```python
from build123d import *

# Parameters (mm, degrees)
SKETCH001_W     = 145.57
SKETCH001_H     = 82.477117
PAD_DEPTH       = 3
PAD001_DEPTH    = 165.3
SKETCH004_W     = 328.820023
SKETCH004_H     = 275.658927
POCKET_DEPTH    = 200
PAD002_DEPTH    = 3
SKETCH003_R     = 1.4
PAD003_DEPTH    = 10
SKETCH005_R     = 7.5
POCKET001_DEPTH = 46.158923


with BuildPart() as part:
    # Sketch001 → Pad (new body)
    with BuildSketch(Plane.XY):
        with Locations((0, 4.919365)):
            Rectangle(SKETCH001_W, SKETCH001_H)
    extrude(amount=-PAD_DEPTH)

    # Sketch → Pad001 (join)
    with BuildSketch(Plane.XY):
        Polygon((51.785, -21.319194), (57.785, -21.319194), (57.785, 31.157923), (-57.785, 31.157923), (-57.785, -21.319194), (-51.785, -21.319194), (-51.785, 25.157923), (51.785, 25.157923), align=None)
    extrude(amount=PAD001_DEPTH)

    # Sketch004 (on DatumPlane) → Pocket (cut)
    with BuildSketch(Plane(origin=(0, -35, 0), x_dir=(1, 0, 0), z_dir=(0, -0.939693, 0.34202))):
        with Locations((-2.626228, 137.829464)):
            Rectangle(SKETCH004_W, SKETCH004_H)
    extrude(amount=POCKET_DEPTH, mode=Mode.SUBTRACT)

    # Sketch002 (on DatumPlane) → Pad002 (join)
    with BuildSketch(Plane(origin=(0, -35, 0), x_dir=(1, 0, 0), z_dir=(0, -0.939693, 0.34202))):
        Polygon((-57.785, 175.89), (57.785, 175.89), (57.785, 40), (51.785, 40), (51.785, 62), (-5.215, 62), (-5.215, 40), (-57.785, 40), align=None)
    extrude(amount=-PAD002_DEPTH)

    # Sketch003 (on DatumPlane) → Pad003 (join)
    with BuildSketch(Plane(origin=(0, -35, 0), x_dir=(1, 0, 0), z_dir=(0, -0.939693, 0.34202))):
        with Locations((-54.61, 172.715)):
            Circle(SKETCH003_R)
        with Locations((54.61, 172.715)):
            Circle(SKETCH003_R)
        with Locations((54.61, 43.175)):
            Circle(SKETCH003_R)
        with Locations((-54.61, 43.175)):
            Circle(SKETCH003_R)
    extrude(amount=PAD003_DEPTH)

    # Sketch005 → Pocket001 (cut, through all)
    with BuildSketch(Plane.XZ):
        with Locations((0, 20)):
            Circle(SKETCH005_R)
    extrude(amount=-POCKET001_DEPTH, mode=Mode.SUBTRACT)


solid = part.part
```
CAD build for the part. Positions are in the model's coordinates, mm. A direction names the side the tool comes from. Coordinates: 2 decimals unless noted, no trailing zeros. Write each loop counter-clockwise with the first axis right and the second up, starting at its lowest first coordinate (ties: lowest second). Pieces come first, ordered by that corner, then holes. Notation, with made-up numbers: (52, -24) -> (60, -24) arc R30 cw to (60, 1) -> close; hole circle Ø6 at (78, 86). An arc over 180 degrees is marked (long way). Use CSV: the item, a comma, the result in double quotes. Start each with the question number.
Item 1: Tool access for faces 4 (the flat face through (-57.785, 11, 63)), 5 (the flat face through (57.785, 10, 63)), 6 (the flat face through (-5.215, -16, 48)), 7 (the flat face through (55, -21.319, 19)), 8 (the flat face through (-51.785, 7, 60)): list every direction of +Z, -Z, +X, -X, +Y, -Y with a clear straight run to the whole face (end or side of a thin tool).
Item 2: Two-plate mould, pull along Z, no slides. Class faces 1 (the flat face through (-1, 25.158, 77)), 2 (the flat face through (-1, 5, -3)), 3 (the flat face through (1, 31.158, 81)): +Z half, -Z half, draft (parallel to the pull), parting line (faces both ways), or undercut.
Item 3: Band-saw the part on A-A, the plane z = 20. Write the cut outline in (x, y) (3 decimals), plus the area to 3 significant figures.
Item 4: Wall check: probe 1 along X at (y, z) = (20, 101.5) (3 decimals); probe 2 along Z at (x, y) = (0, 27); probe 3 along X at (y, z) = (25.5, 119) (3 decimals). Give the ranges that are in metal, low to high.
Item 5: Band-saw the part on D-D, the plane z = 150.5. Write the cut outline in (x, y) (3 decimals).
Item 6: Drop flat-ended pins along their axis: P1, Ø5, axis at x = -56, z = 27.5, coming from the -Y side; P2, Ø3, axis at x = -17.5, y = 34.5, coming from the +Z side; P3, Ø3, axis at y = 2, z = 63.5, coming from the +X side (3 decimals); P4, Ø1, axis at y = -22.5, z = 15, coming from the +X side. Give the stop position or say it passes through.
Response values:
1,face 4,"+Z, -X, +Y, -Y"
1,face 5,"+Z, +X, +Y, -Y"
1,face 6,"-Y"
1,face 7,"+X, -X, -Y"
1,face 8,"none"
2,face 1,"undercut"
2,face 2,"-Z half"
2,face 3,"draft"
3,outline,"(-57.785, -21.319) -> (-51.785, -21.319) -> (-51.785, 25.158) -> (-7.5, 25.158) -> (-7.5, 31.158) -> (-57.785, 31.158) -> close; (7.5, 25.158) -> (51.785, 25.158) -> (51.785, -21.319) -> (57.785, -21.319) -> (57.785, 31.158) -> (7.5, 31.158) -> close"
3,area,"1,160 mm2"
4,probe 1,"x = -57.785 to -51.785, 51.785 to 57.785"
4,probe 2,"z = -3 to 12.5, 27.5 to 165.3"
4,probe 3,"x = -57.785 to 57.785"
5,outline,"(-57.785, 19.777) -> (57.785, 19.777) -> (57.785, 31.158) -> (-57.785, 31.158) -> close; hole (-51.785, 22.97) -> (51.785, 22.97) -> (51.785, 25.158) -> (-51.785, 25.158) -> close"
6,P1,"stops at y = -21.32"
6,P2,"stops at z = 0"
6,P3,"stops at x = 57.785"
6,P4,"passes through"
